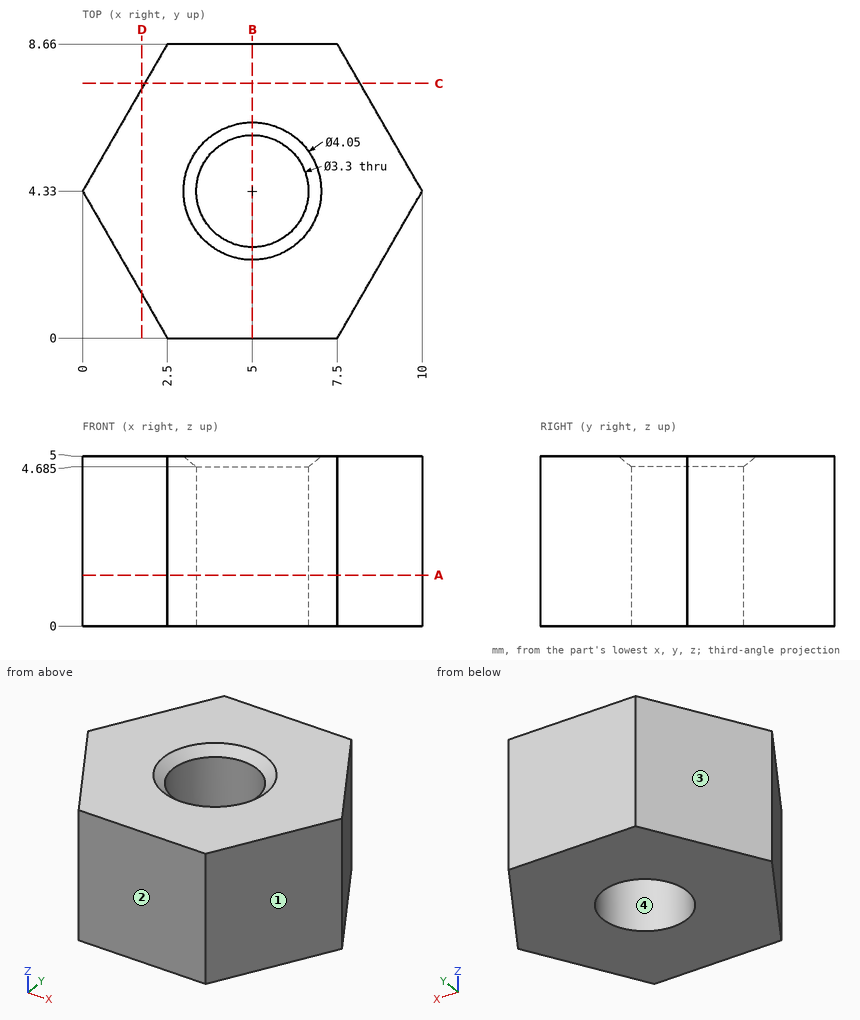
Drawing for the job (mm, zero at the part's lowest x, y, z). Give positions to 0.01 mm unless a question says otherwise; leave off trailing zeros. Order: outer loops, then holes, each group sorted by start corner. A loop starts at its lowest first (then second) coordinate and runs counter-clockwise, first axis right, second up. Notation, with made-up numbers: M -16.5,87.25 L 23.5,87.25 A24 cw 23.5,113.25 Z; hole C 83.5,-40 d8. An arc over 180 degrees is marked long. Use a Markdown table: item, result. Add a question column.
(1) Saw through at A-A, the plane z = 1.5. Give the cut face in (x, y).
(2) Drop a flat-ended pin along its axis: P1, Ø1, axis at y = 1.5, z = 3, coming from the -X side (1 decimal). Give the stop position or say it passes through.
(3) Probe line 1 along Y through (x, z) = (5, 3.25); line 2 along X through (y, z) = (5.25, 1.4); line 3 along X through (y, z) = (3, 2.35) (1 decimal). List the from-to ranges inside material, lowest first. Write a range as [from, to].
(4) Mould opens along X. For the marked faces 1, 2, 3 and 4 say: +X half, -X half, draft (parallel to the pull), parting line (faces both ways), or undercut.
(5) Saw through at D-D, the plane x = 1.75. Give the cut face in (y, z).
(6) Saw through at C-C, the plane y = 7.5. Give the cut face in (x, z).
(7) Saw through at B-B, the plane x = 5. Give the cut face in (y, z) (1 decimal), and give its area (3 significant figures).
Answer key:
| question | item | result |
|---|---|---|
| 1 | outline | M 0,4.33 L 2.5,0 L 7.5,0 L 10,4.33 L 7.5,8.66 L 2.5,8.66 Z; hole C 5,4.33 d3.3 |
| 2 | P1 | x = 1.3 |
| 3 | line 1 | [0, 2.68], [5.98, 8.66] |
| 3 | line 2 | [0.53, 3.63], [6.37, 9.47] |
| 3 | line 3 | [0.8, 4], [6, 9.2] |
| 4 | face 1 | +X half |
| 4 | face 2 | draft |
| 4 | face 3 | -X half |
| 4 | face 4 | undercut |
| 5 | outline | M 1.3,0 L 7.36,0 L 7.36,5 L 1.3,5 Z |
| 6 | outline | M 1.83,0 L 8.17,0 L 8.17,5 L 1.83,5 Z |
| 7 | outline | M 0,0 L 2.7,0 L 2.7,4.7 L 2.3,5 L 0,5 Z; M 6,0 L 8.7,0 L 8.7,5 L 6.4,5 L 6,4.7 Z |
| 7 | area | 26.7 mm^2 |
